Geometry check sheet. Reference: the model listing, model coordinates, mm. Give positions to 0.01 mm unless a question says otherwise; leave off trailing zeros. Loops run counter-clockwise (first coordinate to the right, second up) from the corner with the lowest first, then second, coordinate; pieces in that order, holes last.
Autodesk Inventor part; units mm, degrees
ref_plane "YZ Plane" through (0, 0, 0) normal (1, 0, 0) x (0, 1, 0)
ref_plane "XZ Plane" through (0, 0, 0) normal (0, 1, 0) x (-1, 0, 0)
ref_plane "XY Plane" through (0, 0, 0) normal (0, 0, 1) x (1, 0, 0)
ref_plane "Work Plane1" through (0, 0, 0) normal (0, 0, 1) x (1, 0, 0)
sketch "Sketch1" plane through (0, 0, 0) normal (0, 0, 1) x (1, 0, 0)
  line L0 (0, 0) -> (-101.6, 0)
  line L1 (-101.6, 0) -> (1065.8333, -1167.4333)
  line L2 (1065.8333, -1167.4333) -> (1117.6006, -1219.2006)
  line L3 (1117.6006, -1219.2006) -> (1117.6006, -1117.6006)
  line L4 (1117.6006, -1117.6006) -> (0, 0)
  dimension "d1" = 101.6
  dimension "d2" = 1651
  dimension "d4" = 101.6
extrude "Extrusion1" add sketch "Sketch1" against normal blind 50.8
properties part number "2x4x67.88" material "Wood (Birch)"
1) Sectioned sample at B-B on x = 297.5. Enter the section's corners in (y, z).
2) Depth check by flat-ended pin: P1, Ø4, axis at y = -660, z = -40, coming from the +X side; P2, Ø6, axis at x = 29, z = -25, coming from the +Y side; P3, Ø1.5, axis at x = 638, z = -22.5, coming from the -Y side. Enter the tip coordinate at first touch or a pass-through.
3) Scan lines: line 1 along X through (y, z) = (-403, -36.5); line 2 along X through (y, z) = (-271.5, -21); line 3 along Y through (x, z) = (552.5, -23). Record each from-to range of solid material in increasing order.
4) Sectioned sample at A-A on z = -32.5. Enter the section's corners in (x, y), plus the area to 3 significant figures.
Determined:
1. outline: (-399.1, -50.8) - (-297.5, -50.8) - (-297.5, 0) - (-399.1, 0) - close
2. P1: stops at x = 662
2. P2: stops at y = -26
2. P3: stops at y = -740.35
3. line 1: x = 301.4 to 403
3. line 2: x = 169.9 to 271.5
3. line 3: y = -654.1 to -552.5
4. outline: (-101.6, 0) - (1117.6, -1219.2) - (1117.6, -1117.6) - (0, 0) - close
4. area: 119,000 mm2
